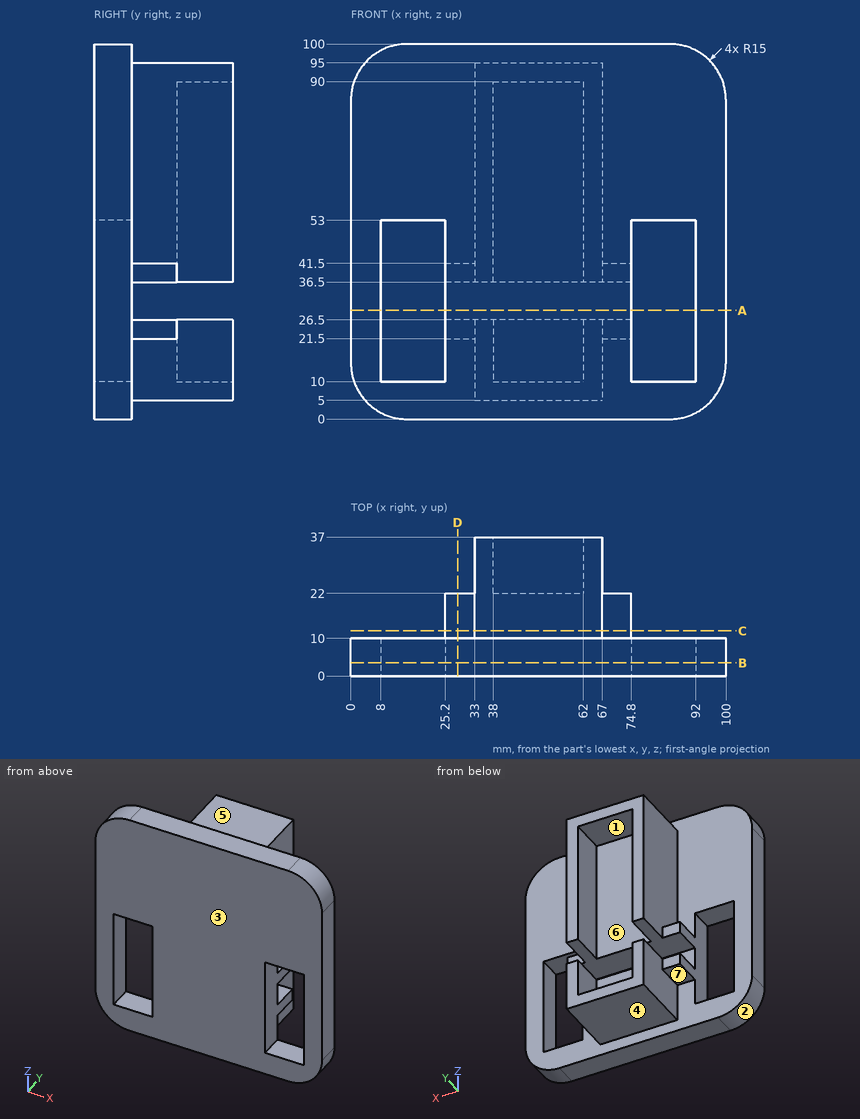
Print and shaded views of the part. All mm, measured from the part's lowest x, y and z. A direction names the side the tool comes from. Coordinates: 2 decimals unless noted, no trailing zeros. Write each loop counter-clockwise with the first axis right and the second up, starting at its lowest first coordinate (ties: lowest second). Pieces come first, ordered by that corner, then holes. Notation, with made-up numbers: (52, -9) - (107, -9) arc R20 cw to (107, 3) - close; hole circle Ø11 at (76, 33.5). An arc over 180 degrees is marked (long way). One line per question, with ' | ' between items. Start each with the question number.
Q1. Drill centre lines: line 1 (X direction, y = 9, z = 23); line 2 (Z direction, x = 47, y = 32.5); line 3 (X direction, y = 27, z = 64.5). Where is each one in solid material? Low to high. Write a range as [from, to].
Q2. 3-axis set-ups, long thin cutter, end or side, ignore diameter. For the marked faces 4, 5, 6 and 7: which of +Z, -Z, +X, -X, +Y, -Y reach the whole face in a straight line?
Q3. Cut at D-D, the plane x = 28.5. List the corners of the cut face in (y, z).
Q4. Cut at A-A, the plane z = 29. List the corners of the cut face in (x, y).
Q5. Cut at C-C, the plane y = 12. List the corners of the cut face in (x, z).
Q6. Pull direction X, two halves, no side cores. Call the marked faces 1, 2 and 3: pulls with the +X half, pulls with the -X half, needs draft (parallel to the pull), parting line crosses it, or undercut.
Q7. Cut at B-B, the plane y = 3.5. List the corners of the cut face in (x, z).
Q8. Pin check, flat tips, straight feed: pin 1 (5 mm diameter, centred on x = 47, z = 16, fed in from +Y); pin 2 (8 mm diameter, centred on y = 17.5, z = 66, fed in from +X); pin 3 (5 mm diameter, centred on x = 64, y = 24, fed in from -Z). Stop position of each tip, or through.
Answer below:
1) line 1: [0, 8], [25.2, 74.8], [92, 100] | line 2: [5, 10], [90, 95] | line 3: [33, 38], [62, 67]
2) face 4: -Z, +X, -X, +Y | face 5: +Z, +X, -X, +Y | face 6: +Y | face 7: -Z, -X, +Y
3) outline: (0, 0) - (10, 0) - (10, 21.5) - (22, 21.5) - (22, 26.5) - (10, 26.5) - (10, 36.5) - (22, 36.5) - (22, 41.5) - (10, 41.5) - (10, 100) - (0, 100) - close
4) outline: (0, 0) - (8, 0) - (8, 10) - (0, 10) - close; (25.2, 0) - (74.8, 0) - (74.8, 10) - (25.2, 10) - close; (92, 0) - (100, 0) - (100, 10) - (92, 10) - close
5) outline: (25.2, 21.5) - (33, 21.5) - (33, 5) - (67, 5) - (67, 21.5) - (74.8, 21.5) - (74.8, 26.5) - (25.2, 26.5) - close; (25.2, 36.5) - (74.8, 36.5) - (74.8, 41.5) - (67, 41.5) - (67, 95) - (33, 95) - (33, 41.5) - (25.2, 41.5) - close
6) face 1: undercut | face 2: pulls with the -X half | face 3: needs draft
7) outline: (0, 15) arc R15 ccw to (15, 0) - (85, 0) arc R15 ccw to (100, 15) - (100, 85) arc R15 ccw to (85, 100) - (15, 100) arc R15 ccw to (0, 85) - close; hole (8, 10) - (25.2, 10) - (25.2, 53) - (8, 53) - close; hole (74.8, 10) - (92, 10) - (92, 53) - (74.8, 53) - close
8) pin 1: y = 22 | pin 2: x = 67 | pin 3: z = 5
